```python
from build123d import *

# Parameters (mm, degrees)
PAD_DEPTH            = 18
SKETCH_R             = 2.6
POCKET_DEPTH         = 339.017224
POCKET_DEPTH_BACK    = 357.017224
SKETCH001_R          = 2.6
POCKET001_DEPTH      = 339.017224
POCKET001_DEPTH_BACK = 357.017224
SKETCH002_R          = 20
POCKET002_DEPTH      = 339.017224
POCKET002_DEPTH_BACK = 357.017224
SKETCH004_R          = 2.7
POCKET003_DEPTH      = 339.017224
POCKET003_DEPTH_BACK = 357.017224
SKETCH005_R          = 2.7
POCKET004_DEPTH      = 339.017224
POCKET004_DEPTH_BACK = 357.017224


with BuildPart() as part:
    # Sketch003 → Pad (new body)
    with BuildSketch(Plane.XY):
        Polygon((0, 92.25), (53, 92.25), (53, -67.75), (0, -67.75), (0, 0), align=None)
    pad = extrude(amount=PAD_DEPTH)

    # Sketch → Pocket (cut, two sides)
    with BuildSketch(Plane(origin=(18, 0, 0), x_dir=(1, 0, 0), z_dir=(0, 0, 1))) as pocket_sk:
        Circle(SKETCH_R)
        with Locations((0, 32)):
            Circle(SKETCH_R)
    pocket = extrude(amount=-POCKET_DEPTH, mode=Mode.SUBTRACT) + extrude(pocket_sk.sketch, amount=POCKET_DEPTH_BACK, mode=Mode.SUBTRACT)

    # Sketch001 → Pocket001 (cut, two sides)
    with BuildSketch(Plane(origin=(15, 55, 0), x_dir=(1, 0, 0), z_dir=(0, 0, 1))) as pocket001_sk:
        Circle(SKETCH001_R)
        with Locations((0, 30)):
            Circle(SKETCH001_R)
    pocket001 = extrude(amount=-POCKET001_DEPTH, mode=Mode.SUBTRACT) + extrude(pocket001_sk.sketch, amount=POCKET001_DEPTH_BACK, mode=Mode.SUBTRACT)

    # Sketch002 → Pocket002 (cut, two sides)
    with BuildSketch(Plane(origin=(0, -39.5, 0), x_dir=(1, 0, 0), z_dir=(0, 0, 1))) as pocket002_sk:
        Circle(SKETCH002_R)
    pocket002 = extrude(amount=-POCKET002_DEPTH, mode=Mode.SUBTRACT) + extrude(pocket002_sk.sketch, amount=POCKET002_DEPTH_BACK, mode=Mode.SUBTRACT)

    # Sketch004 → Pocket003 (cut, two sides)
    with BuildSketch(Plane(origin=(23.5, -39.5, 0), x_dir=(1, 0, 0), z_dir=(0, 0, 1))) as pocket003_sk:
        with Locations((0, 23.5)):
            Circle(SKETCH004_R)
        with Locations((0, -23.5)):
            Circle(SKETCH004_R)
    pocket003 = extrude(amount=-POCKET003_DEPTH, mode=Mode.SUBTRACT) + extrude(pocket003_sk.sketch, amount=POCKET003_DEPTH_BACK, mode=Mode.SUBTRACT)

    # Sketch005 → Pocket004 (cut, two sides)
    with BuildSketch(Plane(origin=(30, 43, 0), x_dir=(1, 0, 0), z_dir=(0, 0, 1))) as pocket004_sk:
        Circle(SKETCH005_R)
    pocket004 = extrude(amount=-POCKET004_DEPTH, mode=Mode.SUBTRACT) + extrude(pocket004_sk.sketch, amount=POCKET004_DEPTH_BACK, mode=Mode.SUBTRACT)

    # Mirrored: Pad, Pocket, Pocket001, Pocket002, Pocket003, Pocket004 across Sketch003 V_Axis
    add(pad.mirror(Plane(origin=(0, 0, 0), x_dir=(0, 0, 1), z_dir=(1, 0, 0))))
    add(pocket.mirror(Plane(origin=(0, 0, 0), x_dir=(0, 0, 1), z_dir=(1, 0, 0))), mode=Mode.SUBTRACT)
    add(pocket001.mirror(Plane(origin=(0, 0, 0), x_dir=(0, 0, 1), z_dir=(1, 0, 0))), mode=Mode.SUBTRACT)
    add(pocket002.mirror(Plane(origin=(0, 0, 0), x_dir=(0, 0, 1), z_dir=(1, 0, 0))), mode=Mode.SUBTRACT)
    add(pocket003.mirror(Plane(origin=(0, 0, 0), x_dir=(0, 0, 1), z_dir=(1, 0, 0))), mode=Mode.SUBTRACT)
    add(pocket004.mirror(Plane(origin=(0, 0, 0), x_dir=(0, 0, 1), z_dir=(1, 0, 0))), mode=Mode.SUBTRACT)


with BuildPart() as part_1:
    # Clone placement: moved
    add(part.part.moved(Location((53, 67.75, 0))))


solid = part_1.part
```
Work out the finished part from the listing and answer in its coordinate system (mm). Give positions to 0.01 mm unless a question says otherwise; leave off trailing zeros. Write each loop counter-clockwise with the first axis right and the second up, starting at its lowest first coordinate (ties: lowest second). Pieces come first, ordered by that corner, then holes. Notation, with made-up numbers: (55, -27) -> (94, -27) arc R19 cw to (94, 0) -> close; hole circle Ø5 at (74, -4.5). An arc over 180 degrees is marked (long way). Write each question's results on one line, items separated by ' | '.
1. Find section C-C on x = 28.5. Determine the outline of the cut face in (y, z).
Data:
outline: (0, 0) -> (2.24, 0) -> (2.24, 18) -> (0, 18) -> close; (7.26, 0) -> (49.24, 0) -> (49.24, 18) -> (7.26, 18) -> close; (54.26, 0) -> (160, 0) -> (160, 18) -> (54.26, 18) -> close
2. Determine the mould class of faces 1 (the flat face through (52, 0, 9)), 2 (the flat face through (0, 81, 9)), 3 (the cylindrical face through (38.56, 150.21, 9.13)), 4 (the cylindrical face through (33.924, 34.257, 9.126)) for opening direction X: +X half, -X half, draft (parallel to the pull), parting line (faces both ways), or undercut.
Data:
face 1: draft | face 2: -X half | face 3: undercut | face 4: undercut
3. Find section A-A on y = 51.75. Determine the outline of the cut face in (x, z).
Data:
outline: (0, 0) -> (26.8, 0) -> (26.8, 18) -> (0, 18) -> close; (32.2, 0) -> (73.8, 0) -> (73.8, 18) -> (32.2, 18) -> close; (79.2, 0) -> (106, 0) -> (106, 18) -> (79.2, 18) -> close
4. Straight lines are drawn through the part: L1, parallel to X at y = 67.75, z = 14; L2, parallel to X at y = 110.75, z = 8.5; L3, parallel to Y at x = 38, z = 10.25. For each, find the intervals that lie inside material, in ascending order.
Data:
L1: 0 to 32.4, 37.6 to 68.4, 73.6 to 106 | L2: 0 to 20.3, 25.7 to 80.3, 85.7 to 106 | L3: 0 to 15.02, 41.48 to 120.15, 125.35 to 150.15, 155.35 to 160
5. Find section B-B on z = 10.75. Give the number of separate pieces and of enclosed holes in the cut face, and give its area (3 significant figures).
Data:
separate pieces: 1 | enclosed holes: 15 | area: 15,400 mm^2
6. This flat-tipped pin is pushed along its axis until it touches: pin 1 Ø6 at (x, y) = (76.5, 4.75) entering from -Z. Where does it stop, or does it pass through?
Data:
pin 1: z = 0
7. Find section D-D on y = 30.5. Determine the outline of the cut face in (x, z).
Data:
outline: (0, 0) -> (33.13, 0) -> (33.13, 18) -> (0, 18) -> close; (72.87, 0) -> (106, 0) -> (106, 18) -> (72.87, 18) -> close
